Part print with two shaded views. Sizes in mm from the minimum x, y, z corner. A direction names the side the tool comes from. Give positions to 0.01 mm unless a question says otherwise; leave off trailing zeros. Write each loop counter-clockwise with the first axis right and the second up, starting at its lowest first coordinate (ties: lowest second). Pieces come first, ordered by that corner, then holes. Notation, with made-up numbers: M 44,73 L 97,73 A17 ccw 97,98 Z; hole C 59.25,48.25 d3. An arc over 180 degrees is marked long. Return JSON: item names as keys, results as strings. Group by question number.
Q1. Flat gauge pins, fed straight in: pin 1 Ø5 at (y, z) = (22, 4) entering from +X; pin 2 Ø5 at (x, z) = (12.5, 17) entering from +Y; pin 3 Ø6 at (x, y) = (26.5, 16) entering from +Z. Where does each tip first touch, or does it go through?
Q2. Band-saw the part on A-A, the plane x = 18. Give the cut face in (y, z), then the cut area to 3 significant figures.
Q3. Wall check: probe 1 along Z at (x, y) = (15.5, 32); probe 2 along Y at (x, z) = (17, 16.5); probe 3 along Y at (x, z) = (44, 9.5). Give the ranges that are in metal, low to high.
Q4. Band-saw the part on D-D, the plane x = 32. Give the cut face in (y, z).
Q5. Band-saw the part on C-C, the plane z = 17. Give the cut face in (x, y).
Q6. Tool access for the marked faces 1, 2 and 3: list every direction of +Z, -Z, +X, -X, +Y, -Y with a clear straight run to the whole face (end or side of a thin tool).
Q7. Pull direction Z, two halves, no side cores. Call the marked faces 4, 5, 6 and 7: +Z half, -Z half, draft (parallel to the pull), parting line (faces both ways), or undercut.
Q8. Band-saw the part on B-B, the plane y = 33.5. Give the cut face in (x, z), then the cut area to 3 significant figures.
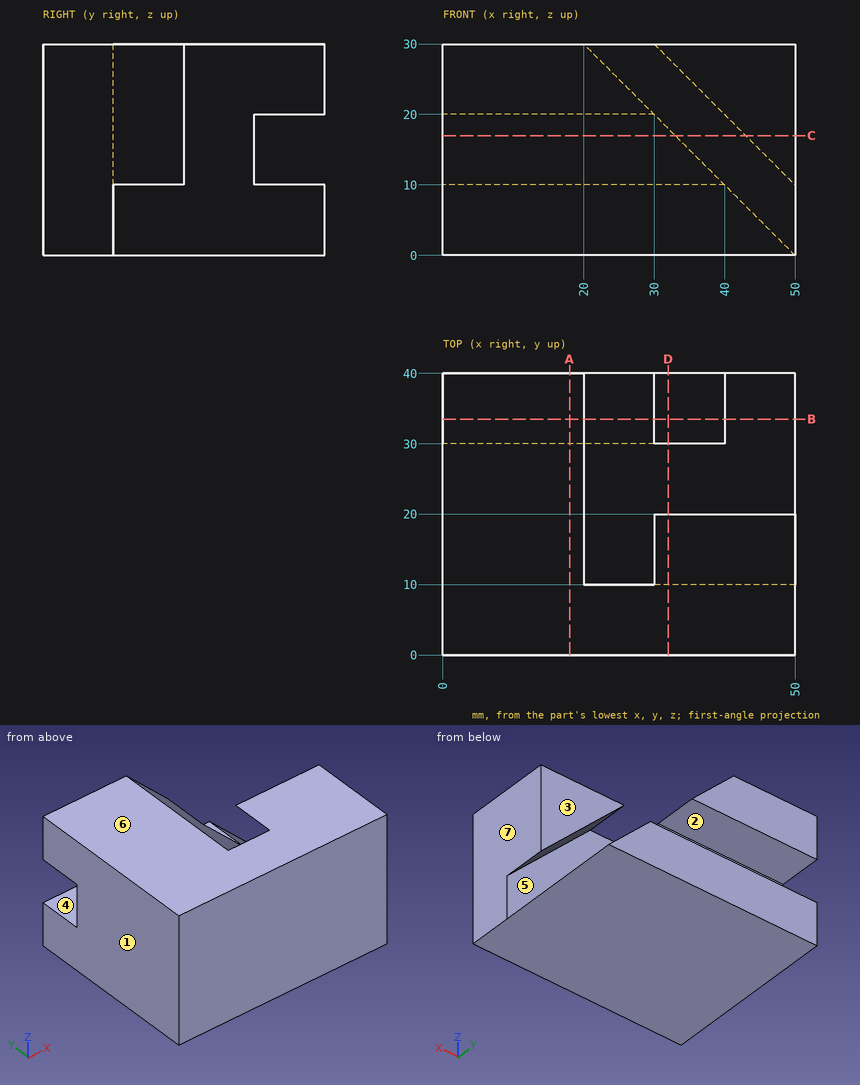
From the geometry:
{
 "1": {"pin 1": "stops at x = 48.5", "pin 2": "stops at y = 30", "pin 3": "stops at z = 26.5"},
 "2": {"outline": "M 0,0 L 40,0 L 40,10 L 30,10 L 30,20 L 40,20 L 40,30 L 0,30 Z", "area": "1,100 mm^2"},
 "3": {"probe 1": "z = 0 to 10, 20 to 30", "probe 2": "y = 0 to 30", "probe 3": "y = 0 to 10"},
 "4": {"outline": "M 0,0 L 40,0 L 40,10 L 30,10 L 30,18 L 10,18 L 10,28 L 20,28 L 20,30 L 0,30 Z"},
 "5": {"outline": "M 0,0 L 50,0 L 50,20 L 43,20 L 43,10 L 33,10 L 33,30 L 0,30 Z"},
 "6": {"face 1": "+Z, -Z, -X, +Y, -Y", "face 2": "+X, -X, +Y", "face 3": "+Z, +X, +Y"},
 "7": {"face 4": "undercut", "face 5": "undercut", "face 6": "+Z half", "face 7": "draft"},
 "8": {"outline": "M 0,0 L 50,0 L 40,10 L 0,10 Z; M 0,20 L 30,20 L 20,30 L 0,30 Z", "area": "700 mm^2"}
}
